Input: dimensioned drawing with shaded views. Units: mm. Origin: part minimum x, y, z. Give positions to 0.01 mm unless a question says otherwise; leave off trailing zeros. Loops run counter-clockwise (first coordinate to the right, second up) from the corner with the lowest first, then second, coordinate; pieces in that order, holes last. Notation, with made-up numbers: M 6.25,-33 L 48.25,-33 A33 ccw 48.25,3 Z; hole C 64.25,45.5 d8. An arc over 180 degrees is marked long. Answer in a Markdown table with one row per item.
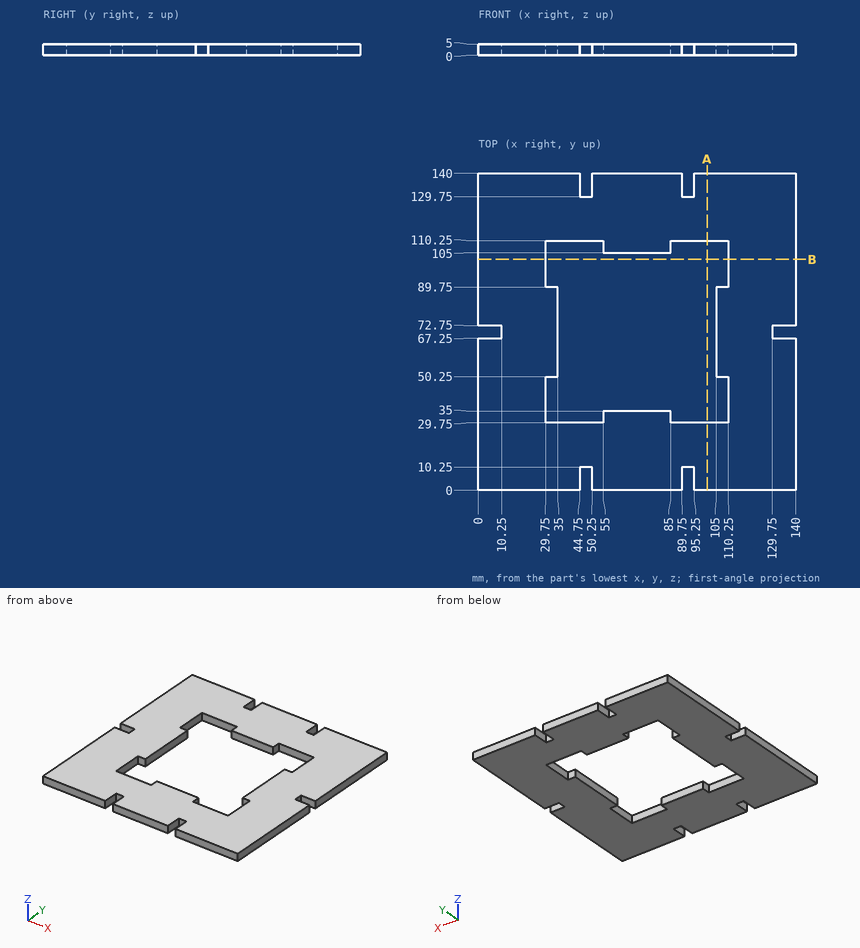
Q1. Section query A-A (x = 101). Output: boundary loops of the cut face in (y, z).
Values follow:
| item | result |
|---|---|
| outline | M 0,0 L 29.75,0 L 29.75,5 L 0,5 Z; M 110.25,0 L 140,0 L 140,5 L 110.25,5 Z |
Q2. Ray query, probe 1 along X at (y, z) = (109.5, 1.15); probe 2 along Y at (x, z) = (45.5, 2.9); probe 3 along Y at (x, z) = (41, 0.35). Return the intervals inside material, ascending. Write a range as from..to.
Values follow:
| item | result |
|---|---|
| probe 1 | 0..29.75, 55..85, 110.25..140 |
| probe 2 | 10.25..29.75, 110.25..129.75 |
| probe 3 | 0..29.75, 110.25..140 |
Q3. Contact query for flat-ended pins moving along their axis: pin 1 Ø1 at (x, z) = (17, 1) entering from -Y; pin 2 Ø1.5 at (x, z) = (48.5, 3) entering from +Y; pin 3 Ø1 at (y, z) = (68, 3.5) entering from +X; pin 4 Ø1.5 at (x, z) = (92, 2) entering from -Y. Output: stop coordinate, or through.
Values follow:
| item | result |
|---|---|
| pin 1 | y = 0 |
| pin 2 | y = 129.75 |
| pin 3 | x = 129.75 |
| pin 4 | y = 10.25 |
